Design review of the part shown in the three views and the two pictorial views. Dimensions are in mm from the part's minimum x, y and z. Round coordinates to 2 decimals unless told otherwise and drop trailing zeros. Write each loop counter-clockwise with the first axis right and the second up, starting at its lowest first coordinate (ties: lowest second). Pieces come first, ordered by that corner, then holes. Notation, with made-up numbers: (-27, -31) -> (-7, -31) arc R22 ccw to (-7, -8) -> close; hole circle Ø4 at (83, 41.5). An arc over 180 degrees is marked (long way). One line per question, with ' | ' between items. Start each with the question number.
1) Consider section B-B (x = 161). Give the boundary of the cut face in (y, z) (1 decimal).
2) Insertion check: pin 1 Ø0.5 at (x, y) = (115, 1) entering from -Z; pin 2 Ø1.3 at (x, y) = (98, 1) entering from -Z. Each pin has a flat end and moves straight along its axis. Give the tip position at first contact, or say it passes through.
3) For probe 1 along X at (y, z) = (0.25, 30) (1 decimal); probe 2 along Z at (x, y) = (91, 0.65); probe 3 along X at (y, z) = (1.25, 24.5), list the stretches that pass through material, from the lowest coordinate up.
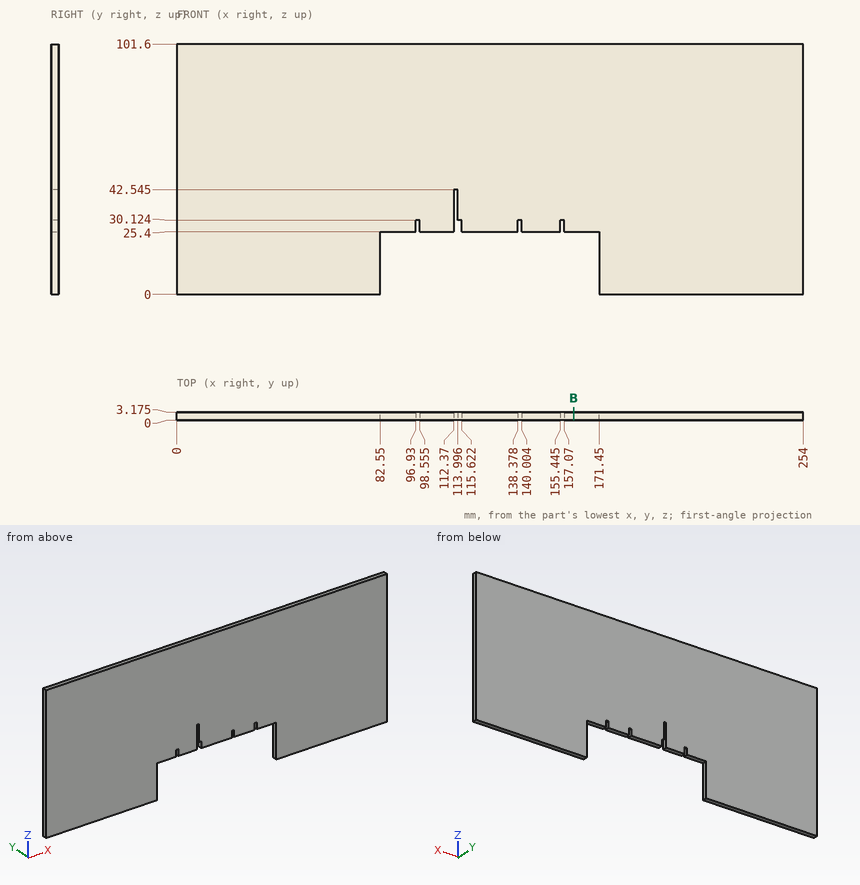
From the geometry:
1) outline: (0, 25.4) -> (3.2, 25.4) -> (3.2, 101.6) -> (0, 101.6) -> close
2) pin 1: stops at z = 30.12 | pin 2: stops at z = 25.4
3) probe 1: x = 0 to 96.9, 98.6 to 112.4, 115.6 to 138.4, 140 to 155.4, 157.1 to 254 | probe 2: z = 25.4 to 101.6 | probe 3: x = 0 to 82.55, 171.45 to 254
